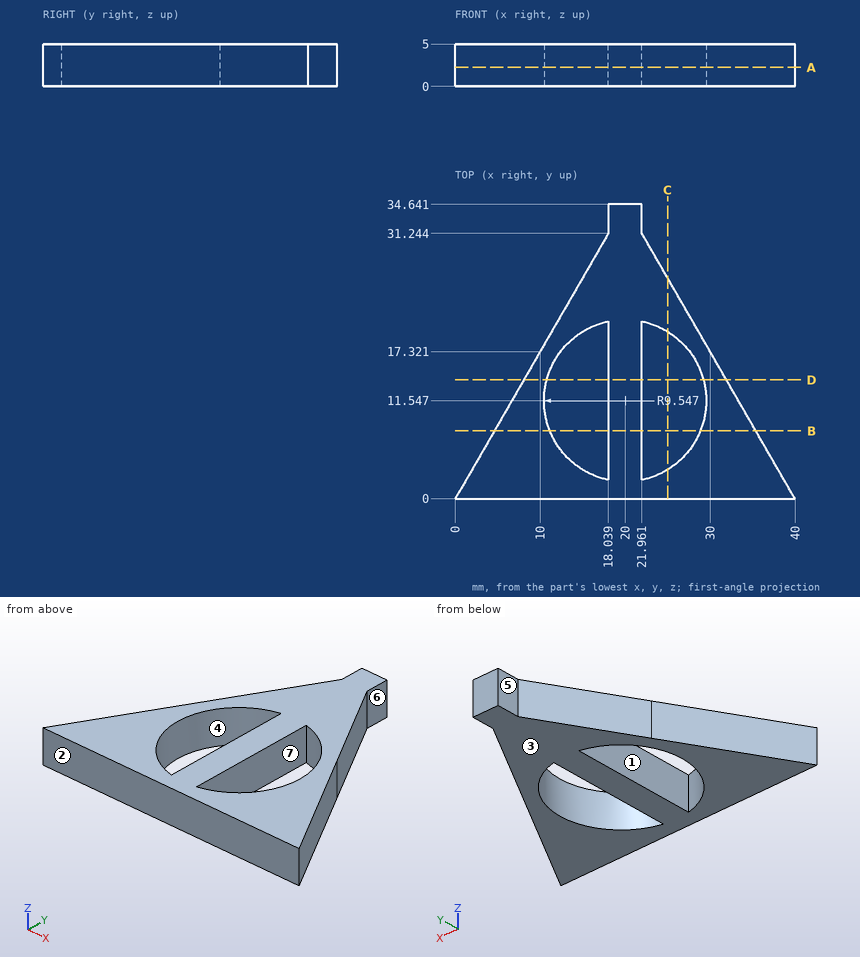
Print and shaded views of the part. All mm, measured from the part's lowest x, y and z. A direction names the side the tool comes from. Coordinates: 2 decimals unless noted, no trailing zeros. Order: outer loops, then holes, each group sorted by start corner. A loop starts at its lowest first (then second) coordinate and runs counter-clockwise, first axis right, second up. Notation, with made-up numbers: (7, 8) - (65, 8) arc R9 cw to (65, 14) - close; hole circle Ø8 at (81.25, 76). An arc over 180 degrees is marked (long way). Return JSON: item names as keys, results as strings. Group by question number.
Item 1: Cut at C-C (x = 25). List the corners of the cut face in (y, z) (1 decimal).
Item 2: Drill centre lines: probe 1 along X at (y, z) = (10, 2.45) (1 decimal); probe 2 along X at (y, z) = (15, 2.85); probe 3 along X at (y, z) = (33.5, 3.35). Where is each one in solid material? Low to high. Write a range as from..to.
Item 3: Cut at B-B (y = 8). List the corners of the cut face in (x, z).
Item 4: Cut at D-D (y = 14). List the corners of the cut face in (x, z).
Item 5: Pin check, flat tips, straight feed: pin 1 (2 mm diameter, centred on x = 30, y = 20, fed in from -Z); pin 2 (2.5 mm diameter, centred on y = 33, z = 3, fed in from +X); pin 3 (2.5 mm diameter, centred on y = 15.5, z = 2.5, fed in from +X); pin 4 (1 mm diameter, centred on y = 19.5, z = 2.5, fed in from -X). Stop position of each tip, or through.
Item 6: Which spindle directions (+Z, -Z, +X, -X, +Y, -Y) get a long thin tool onto all of the face, cutting with end or side? Do the marked faces 5, 6 and 7. Say none if no direction does.
Item 7: Pull direction Y, two halves, no side cores. Call the marked faces 1, 2, 3 and 4: pulls with the +Y half, pulls with the -Y half, needs draft (parallel to the pull), parting line crosses it, or undercut.
Item 8: Cut at A-A (z = 2.25). List the corners of the cut face in (x, y) (1 decimal).
Check values:
{
 "1": {"outline": "(0, 0) - (3.4, 0) - (3.4, 5) - (0, 5) - close; (19.7, 0) - (26, 0) - (26, 5) - (19.7, 5) - close"},
 "2": {"probe 1": "x = 5.8..10.6, 18..22, 29.4..34.2", "probe 2": "x = 8.66..11.1, 18.04..21.96, 28.9..31.34", "probe 3": "x = 18.04..21.96"},
 "3": {"outline": "(4.62, 0) - (11.14, 0) - (11.14, 5) - (4.62, 5) - close; (18.04, 0) - (21.96, 0) - (21.96, 5) - (18.04, 5) - close; (28.86, 0) - (35.38, 0) - (35.38, 5) - (28.86, 5) - close"},
 "4": {"outline": "(8.08, 0) - (10.77, 0) - (10.77, 5) - (8.08, 5) - close; (18.04, 0) - (21.96, 0) - (21.96, 5) - (18.04, 5) - close; (29.23, 0) - (31.92, 0) - (31.92, 5) - (29.23, 5) - close"},
 "5": {"pin 1": "passes through", "pin 2": "stops at x = 21.96", "pin 3": "stops at x = 31.77", "pin 4": "stops at x = 10.97"},
 "6": {"face 5": "+Z, -Z, -X, +Y", "face 6": "+Z, -Z, +X, +Y", "face 7": "+Z, -Z"},
 "7": {"face 1": "undercut", "face 2": "pulls with the -Y half", "face 3": "needs draft", "face 4": "undercut"},
 "8": {"outline": "(0, 0) - (40, 0) - (22, 31.2) - (22, 34.6) - (18, 34.6) - (18, 31.2) - close; hole (18, 2.2) - (18, 20.9) arc R9.5 ccw to start; hole (22, 2.2) arc R9.5 ccw to (22, 20.9) - close"}
}
